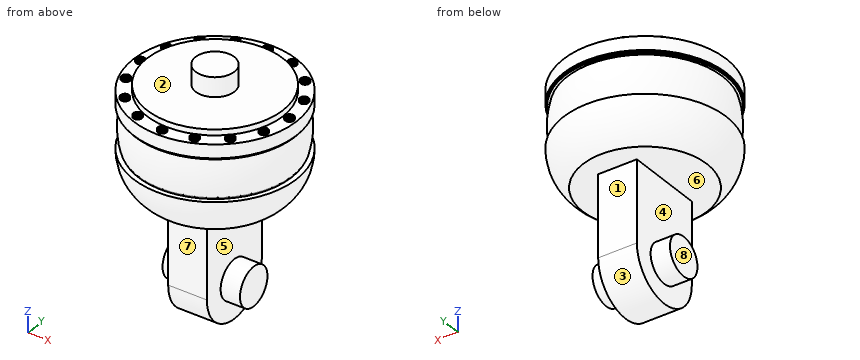
from build123d import *

# Parameters (mm, degrees)
SKETCH2_R           = 39.5
BOSS_EXTRUDE1_DEPTH = 1
SKETCH4_R           = 41.25
BOSS_EXTRUDE2_DEPTH = 1
SKETCH5_R           = 42
BOSS_EXTRUDE3_DEPTH = 7
SKETCH6_R           = 35
BOSS_EXTRUDE4_DEPTH = 3
SKETCH7_R           = 2.25
SKETCH7_R_2         = 1.5
BOSS_EXTRUDE5_DEPTH = 1
CIRPATTERN1_COUNT   = 16
SKETCH8_W           = 20
SKETCH8_H           = 40
BOSS_EXTRUDE6_DEPTH = 42
SKETCH9_R           = 20
BOSS_EXTRUDE7_DEPTH = 20
SKETCH10_R          = 10
BOSS_EXTRUDE8_DEPTH = 10
SKETCH11_R          = 10
BOSS_EXTRUDE9_DEPTH = 10


with BuildPart() as part:
    # Sketch1 → Revolve1 (revolve)
    with BuildSketch(Plane(origin=(0, 0, 0), x_dir=(1, 0, 0), z_dir=(0, 1, 0))):
        with BuildLine():
            Line((0, 0), (0, -20))
            Line((0, -20), (-42, -20))
            ThreePointArc((-42, -20), (-39.360679775, -8.819660113), (-32, 0))
            Line((-32, 0), (0, 0))
        make_face()
    revolve(axis=Axis((0, 0, 0), (0, 0, 1)))

    # Sketch2 → Boss-Extrude1 (add)
    with BuildSketch(Plane.XY.offset(20)):
        Circle(SKETCH2_R)
    extrude(amount=BOSS_EXTRUDE1_DEPTH)

    # Sketch3 → Revolve2 (revolve)
    with BuildSketch(Plane(origin=(0, 0, 0), x_dir=(1, 0, 0), z_dir=(0, 1, 0))):
        with BuildLine():
            Line((0, -21), (-40, -21))
            ThreePointArc((-40, -21), (-41.376973739, -31), (-40, -41))
            Line((-40, -41), (0, -41))
            Line((0, -41), (0, -21))
        make_face()
    revolve(axis=Axis((0, 0, 21), (0, 0, 1)))

    # Sketch4 → Boss-Extrude2 (add)
    with BuildSketch(Plane.XY.offset(41)):
        Circle(SKETCH4_R)
    extrude(amount=BOSS_EXTRUDE2_DEPTH)

    # Sketch5 → Boss-Extrude3 (add)
    with BuildSketch(Plane.XY.offset(42)):
        Circle(SKETCH5_R)
    extrude(amount=BOSS_EXTRUDE3_DEPTH)

    # Sketch6 → Boss-Extrude4 (add)
    with BuildSketch(Plane.XY.offset(49)):
        Circle(SKETCH6_R)
    extrude(amount=BOSS_EXTRUDE4_DEPTH)

    # Sketch7 → Boss-Extrude5 (add)
    with BuildSketch(Plane.XY.offset(49)):
        with Locations((38.5, 0)):
            Circle(SKETCH7_R)
        with Locations((38.5, 0)):
            Circle(SKETCH7_R_2, mode=Mode.SUBTRACT)
    boss_extrude5 = extrude(amount=BOSS_EXTRUDE5_DEPTH)

    # CirPattern1: Boss-Extrude5 ×16 about axis
    cirpattern1_axis = Axis((0, 0, 0), (0, 0, 1))
    for i in range(1, CIRPATTERN1_COUNT):
        add(boss_extrude5.rotate(cirpattern1_axis, i * 360 / CIRPATTERN1_COUNT))

    # Sketch8 → Boss-Extrude6 (add)
    with BuildSketch(Plane(origin=(0, 0, 0), x_dir=(-1, 0, 0), z_dir=(0, 0, -1))):
        Rectangle(SKETCH8_W, SKETCH8_H)
    extrude(amount=BOSS_EXTRUDE6_DEPTH)

    # Sketch9 → Boss-Extrude7 (add)
    with BuildSketch(Plane.ZY.offset(10)):
        with Locations((-42, 0)):
            Circle(SKETCH9_R)
    extrude(amount=-BOSS_EXTRUDE7_DEPTH)

    # Sketch10 → Boss-Extrude8 (add)
    with BuildSketch(Plane.ZY.offset(10)):
        with Locations(Location((-42, 0, 0), (0, 0, 90))):
            Circle(SKETCH10_R)
    boss_extrude8 = extrude(amount=BOSS_EXTRUDE8_DEPTH)

    # Sketch11 → Boss-Extrude9 (add)
    with BuildSketch(Plane.XY.offset(52)):
        Circle(SKETCH11_R)
    extrude(amount=BOSS_EXTRUDE9_DEPTH)

    # Mirror1: Boss-Extrude8 across plane
    add(boss_extrude8.mirror(Plane(origin=(0, 0, 0), x_dir=(0, 0, 1), z_dir=(1, 0, 0))))


solid = part.part
Geometry check sheet. Reference: the model listing, model coordinates, mm. Face numbers are marked on the shaded views. A direction names the side the tool comes from. Give positions to 0.01 mm unless a question says otherwise; leave off trailing zeros. Answer in a Markdown table with one row per item. Add a question column.
1) Material ranges on probe 1 along X at (y, z) = (38.5, 49.75); probe 2 along X at (y, z) = (-14, -15); probe 3 along Y at (x, z) = (5, -26), recorded low to high. Write a range as from..to.
2) Set-up check for the marked faces 5, 6, 7 and 8: record each of +Z, -Z, +X, -X, +Y, -Y from which the full face is reachable in a straight line by a thin tool's end or side.
3) Draft check along Z on the marked faces 1, 2, 3 and 4. Enter one of: pulls with the +Z half, pulls with the -Z half, needs draft (parallel to the pull), parting line crosses it, or undercut.
4) Gauge pin test, flat ends, axial feed: P1, Ø3.5, axis at x = 38, y = 0.5, coming from the +Z side; P2, Ø1.5, axis at x = -15, y = -35, coming from the +Z side; P3, Ø3, axis at x = -14, z = -38, coming from the -Y side. Record the tip position at first contact, or that the pin passes through.
Outcome:
| question | item | result |
|---|---|---|
| 1 | probe 1 | x = -2.25..-1.5, 1.5..2.25 |
| 1 | probe 2 | x = -10..10 |
| 1 | probe 3 | y = -20..20 |
| 2 | face 5 | +X |
| 2 | face 6 | none |
| 2 | face 7 | -Z, +X, -X, -Y |
| 2 | face 8 | -Z, -X, +Y, -Y |
| 3 | face 1 | needs draft |
| 3 | face 2 | pulls with the +Z half |
| 3 | face 3 | pulls with the -Z half |
| 3 | face 4 | undercut |
| 4 | P1 | stops at z = 50 |
| 4 | P2 | stops at z = 49 |
| 4 | P3 | stops at y = -9.68 |
